Study the drawing (mm; zero at the part's minimum x, y, z) and answer. A direction names the side the tool comes from. Coordinates: 2 decimals unless noted, no trailing zeros. Write each loop counter-clockwise with the first axis right and the second up, starting at its lowest first coordinate (ties: lowest second). Pieces come first, ordered by that corner, then holes. Notation, with made-up numbers: M -39,6.25 L -29,6.25 A5 cw -29,13.25 Z; hole C 58,1 d10. An arc over 180 degrees is marked long. Answer as a JSON object with one key per item and string values. Group by question number.
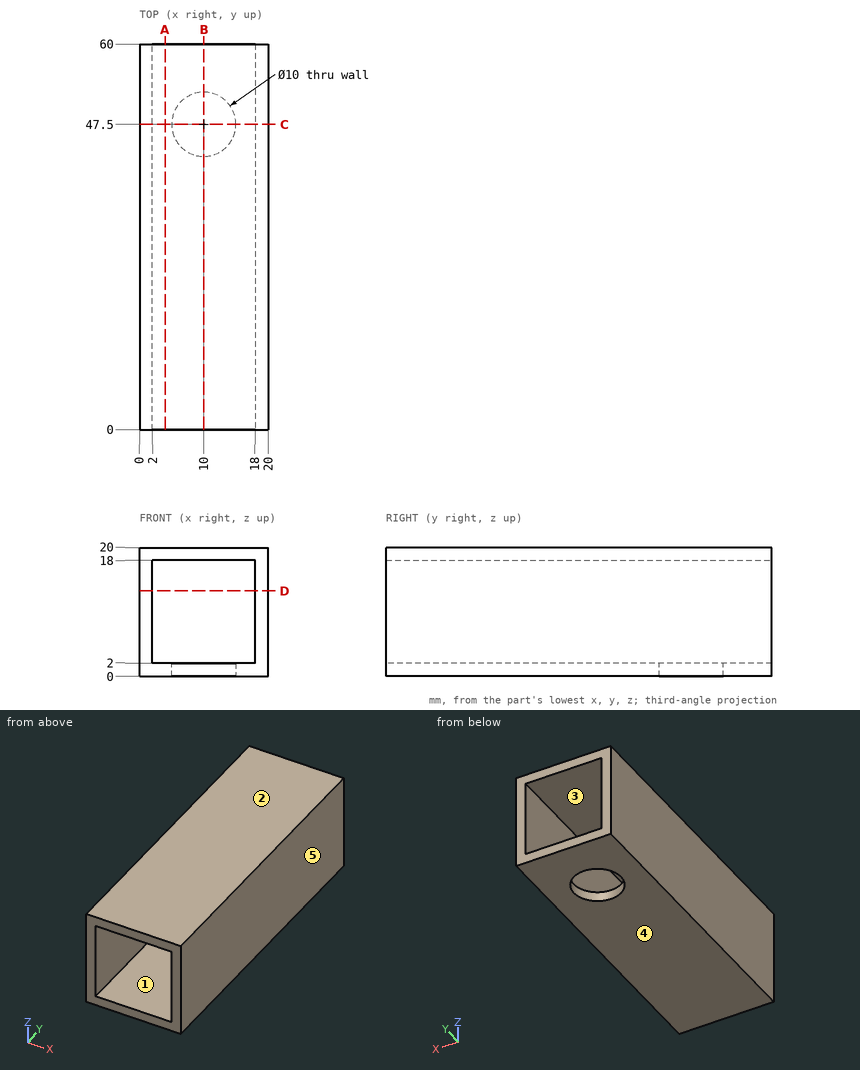
Item 1: Consider L1, parallel to Z at x = 7, y = 9; L2, parallel to Y at x = 10, z = 1.05. Determine where each line is inside the solid, lowest interval first. Write a range as from..to.
Item 2: For a pull along X with two mould halves and no side action, classify the marked faces 3, 4 and 5 as +X half, -X half, draft (parallel to the pull), parting line (faces both ways), or undercut.
Item 3: A cutting plane is placed at B-B, the plane x = 10. Write down the section's boundary in (y, z).
Item 4: A tool of negligible diameter and unlimited length cuts with its end or side. For the marked faces 1 and 2, from which of +Z, -Z, +X, -X, +Y, -Y can it reach the whole face along a straight path? Write none if from no direction.
Item 5: A cutting plane is placed at C-C, the plane y = 47.5. Write down the section's boundary in (x, z), and give its area (3 significant figures).
Item 6: A cutting plane is placed at D-D, the plane z = 13.25. Write down the section's boundary in (x, y), and give its area (3 significant figures).
Item 7: A flat-ended cylindrical pin translates along its axis: pin 1 Ø9 at (x, y) = (10, 47.5) entering from -Z. Find the tip coordinate at first contact, or state that the pin passes through.
Item 8: A cutting plane is placed at A-A, the plane x = 4. Write down the section's boundary in (y, z), and give its area (3 significant figures).
Answer:
{
 "1": {"L1": "0..2, 18..20", "L2": "0..42.5, 52.5..60"},
 "2": {"face 3": "undercut", "face 4": "draft", "face 5": "+X half"},
 "3": {"outline": "M 0,0 L 42.5,0 L 42.5,2 L 0,2 Z; M 0,18 L 60,18 L 60,20 L 0,20 Z; M 52.5,0 L 60,0 L 60,2 L 52.5,2 Z"},
 "4": {"face 1": "+Y, -Y", "face 2": "+Z, +X, -X, +Y, -Y"},
 "5": {"outline": "M 0,0 L 5,0 L 5,2 L 2,2 L 2,18 L 18,18 L 18,2 L 15,2 L 15,0 L 20,0 L 20,20 L 0,20 Z", "area": "124 mm2"},
 "6": {"outline": "M 0,0 L 2,0 L 2,60 L 0,60 Z; M 18,0 L 20,0 L 20,60 L 18,60 Z", "area": "240 mm2"},
 "7": {"pin 1": "z = 18"},
 "8": {"outline": "M 0,0 L 60,0 L 60,2 L 0,2 Z; M 0,18 L 60,18 L 60,20 L 0,20 Z", "area": "240 mm2"}
}
